Verification items for this drawing (mm, ordinates from the low corner). A direction names the side the tool comes from. Coordinates: 2 decimals unless noted, no trailing zeros. Order: outer loops, then holes, each group sorted by start corner. A loop starts at its lowest first (then second) coordinate and runs counter-clockwise, first axis right, second up. Notation, with made-up numbers: (0.25, -10) - (28.25, -10) arc R25 ccw to (28.25, 2) - close; hole circle Ø2 at (54, 57). An arc over 180 degrees is marked (long way). Use CSV: the item, a comma, the result in double quotes. Start each with the question number.
1) Depth check by flat-ended pin: P1, Ø2.5, axis at y = 9, z = 3.5, coming from the -X side; P2, Ø10, axis at x = 21, y = 7, coming from the -Z side; P3, Ø6.5, axis at x = 22, y = 6.5, coming from the -Z side. Enter the tip coordinate at first touch or a pass-through.
2) Thickness scan on probe 1 along Y at (x, z) = (19.05, 23); probe 2 along Z at (x, y) = (9.5, 2.5) (1 decimal); probe 3 along X at (y, z) = (11.25, 4) (1 decimal). Record the ranges inside material, lowest first. Write a range as [from, to].
3) Draft check along X on the marked faces 1, 2 and 3. Enter one of: released by +X, released by -X, zero draft, split by the parting line, or undercut.
4) Sectioned sample at A-A, the plane z = 4. Record the cut outline in (x, y) (1 decimal).
5) Tool access check on the marked faces 4, 5, 6 and 7. Record the directions out of +Z, -Z, +X, -X, +Y, -Y that give a thin tool (end or side, any length) a straight path to the whole face; none if there is none.
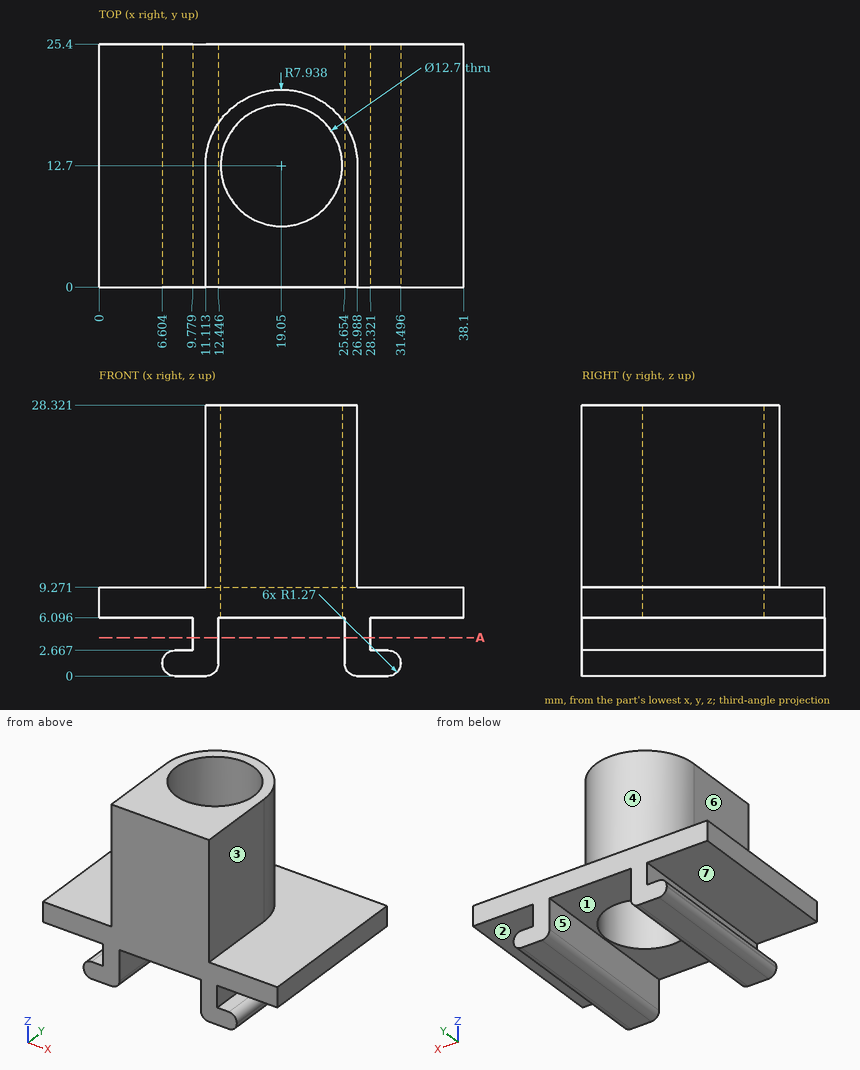
Evaluation:
1,P1,"x = 6.93"
1,P2,"z = 0.4"
1,P3,"z = 6.1"
2,probe 1,"[0, 6.35], [19.05, 20.64]"
2,probe 2,"[0, 2.7], [6.1, 9.3]"
2,probe 3,"[9.8, 12.4], [25.7, 28.3]"
3,face 1,"undercut"
3,face 2,"zero draft"
3,face 3,"released by +X"
4,outline,"(9.8, 0) - (12.4, 0) - (12.4, 25.4) - (9.8, 25.4) - close; (25.7, 0) - (28.3, 0) - (28.3, 25.4) - (25.7, 25.4) - close"
5,face 4,"+Z, +Y"
5,face 5,"-Z, +Y, -Y"
5,face 6,"+Z, -X, +Y, -Y"
5,face 7,"-X, +Y, -Y"
